Can you work these out from the model? Positions are in its coordinate system, mm. Face numbers are marked on the shaded views. A direction names the side the tool comes from. Coordinates: 2 decimals unless noted, no trailing zeros. Loops run counter-clockwise (first coordinate to the right, second up) from the corner with the lowest first, then second, coordinate; pieces in that order, holes last. Notation, with made-up numbers: (20.25, 55.25) -> (42.25, 55.25) arc R11 ccw to (42.25, 64.25) -> close; hole circle Ø8 at (61.25, -8.5). An arc over 180 degrees is marked (long way). Put each result on its own line as item: value. Start each with the question number.
Item 1: If we section it at B-B on y = 1.5: Please give me the cut outline in (x, z).
Item 2: If we section it at A-A on z = -4: Please give me the cut outline in (x, y), plus the area to 3 significant figures.
Item 3: We'd pull the mould along X, two halves only. Please class the marked faces 1, 2 and 3: pulls with the +X half, pulls with the -X half, needs draft (parallel to the pull), parting line crosses it, or undercut.
Item 4: If we section it at C-C on x = 22.25: Please give me the cut outline in (y, z).
Item 5: Will these pins go through, and if not, where does the flat tip stop? P1, Ø1.5, axis at x = 36, y = 5.5, coming from the +Z side; P2, Ø5.5, axis at x = 21, z = -50.5, coming from the +Y side; P3, Ø4, axis at x = 22.25, z = -52.6, coming from the +Y side.
Item 6: If we section it at D-D on y = 8.75: Please give me the cut outline in (x, z).
Item 7: Please list where these lines run through material, in increasing order: L1, parallel to Z at x = 22.25, y = 1.35; L2, parallel to X at y = 1.75, z = -52.6; L3, parallel to Z at x = 22, y = 15.75. Write a range as from..to.
Item 8: For the marked faces 4 and 5, which set-ups out of +Z, -Z, +X, -X, +Y, -Y let a thin tool reach every point of the face, with its end or its side?
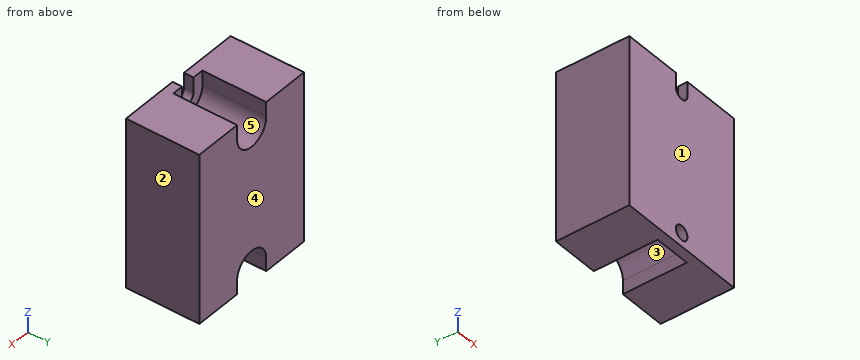
```python
from build123d import *

# Parameters (mm, degrees)
SKETCH1_R           = 2.45
BOSS_EXTRUDE1_DEPTH = 3.2
BOSS_EXTRUDE2_DEPTH = 21.5


with BuildPart() as part:
    # Sketch1 → Boss-Extrude1 (new body)
    with BuildSketch(Plane(origin=(0, 0, 0), x_dir=(1, 0, 0), z_dir=(0, 1, 0))):
        with BuildLine():
            Line((0, 0), (19.8, 0))
            Line((19.8, 0), (19.8, 5))
            ThreePointArc((19.8, 5), (22.25, 7.45), (24.7, 5))
            Line((24.7, 5), (24.7, 0))
            Line((24.7, 0), (44.5, 0))
            Line((44.5, 0), (44.5, 57.2))
            Line((44.5, 57.2), (28.45, 57.2))
            Line((28.45, 57.2), (16.05, 57.2))
            Line((16.05, 57.2), (0, 57.2))
            Line((0, 57.2), (0, 0))
        make_face()
        with Locations((22.25, 52.6)):
            Circle(SKETCH1_R, mode=Mode.SUBTRACT)
    extrude(amount=BOSS_EXTRUDE1_DEPTH)

    # Sketch2 → Boss-Extrude2 (add)
    with BuildSketch(Plane(origin=(0, 3.2, 0), x_dir=(1, 0, 0), z_dir=(0, 1, 0))):
        with BuildLine():
            Line((0, 0), (0, 57.2))
            Line((0, 57.2), (16.05, 57.2))
            Line((16.05, 57.2), (16.05, 52.6))
            ThreePointArc((16.05, 52.6), (22.25, 46.4), (28.45, 52.6))
            Line((28.45, 52.6), (28.45, 57.2))
            Line((28.45, 57.2), (44.5, 57.2))
            Line((44.5, 57.2), (44.5, 0))
            Line((44.5, 0), (28.45, 0))
            Line((28.45, 0), (28.45, 5))
            ThreePointArc((28.45, 5), (22.25, 11.2), (16.05, 5))
            Line((16.05, 5), (16.05, 0))
            Line((16.05, 0), (0, 0))
        make_face()
    extrude(amount=BOSS_EXTRUDE2_DEPTH)


solid = part.part
```
Solutions:
1. outline: (0, -57.2) -> (44.5, -57.2) -> (44.5, 0) -> (24.7, 0) -> (24.7, -5) arc R2.45 cw to (19.8, -5) -> (19.8, 0) -> (0, 0) -> close; hole circle Ø4.9 at (22.25, -52.6)
2. outline: (0, 0) -> (19.8, 0) -> (19.8, 3.2) -> (16.05, 3.2) -> (16.05, 24.7) -> (0, 24.7) -> close; (24.7, 0) -> (44.5, 0) -> (44.5, 24.7) -> (28.45, 24.7) -> (28.45, 3.2) -> (24.7, 3.2) -> close
2. area: 817 mm^2
3. face 1: needs draft
3. face 2: pulls with the +X half
3. face 3: undercut
4. outline: (0, -57.2) -> (3.2, -57.2) -> (3.2, -55.05) -> (0, -55.05) -> close; (0, -50.15) -> (3.2, -50.15) -> (3.2, -46.4) -> (24.7, -46.4) -> (24.7, -11.2) -> (3.2, -11.2) -> (3.2, -7.45) -> (0, -7.45) -> close
5. P1: z = 0
5. P2: y = 3.2
5. P3: through
6. outline: (0, -57.2) -> (16.05, -57.2) -> (16.05, -52.6) arc R6.2 cw to (28.45, -52.6) -> (28.45, -57.2) -> (44.5, -57.2) -> (44.5, 0) -> (28.45, 0) -> (28.45, -5) arc R6.2 cw to (16.05, -5) -> (16.05, 0) -> (0, 0) -> close
7. L1: -57.2..-55.05, -50.15..-7.45
7. L2: 0..19.8, 24.7..44.5
7. L3: -46.41..-11.19
8. face 4: +Z, -Z, +X, -X, +Y
8. face 5: +Z, +Y
